Work out the finished part from the listing and answer in its coordinate system (mm). Face numbers are marked on the shaded views. A direction names the side the tool comes from. Coordinates: 2 decimals unless noted, no trailing zeros. Order: outer loops, then holes, each group sorted by start corner. A loop starts at its lowest first (then second) coordinate and runs counter-clockwise, first axis right, second up. Notation, with made-up numbers: M 81.5,9.25 L 99.5,9.25 A32 ccw 99.5,42.25 Z; hole C -20,67 d4. An arc over 180 degrees is marked long. Use a Markdown table: item, result. Add a question column.
from build123d import *

# Parameters (mm, degrees)
PAD006_DEPTH       = 6.8
POCKET007_DEPTH    = 2.101
POCKET009_DEPTH    = 2.101
CHAMFER003_SIZE    = 0.5
SKETCH023_R        = 3.125
SKETCH023_R_2      = 2
POCKET021_DEPTH    = 2.9
POCKET021_FACE36_R = 3.125
POCKET022_DEPTH    = 3.901
POCKET023_DEPTH    = 5.6
CHAMFER006_SIZE    = 0.4
SKETCH021_R        = 0.5
POCKET024_DEPTH    = 6.801
CHAMFER007_SIZE    = 1


with BuildPart() as part:
    # ShapeBinder001 → Pad006 (new body)
    with BuildSketch(Plane(origin=(0, 0, -2.55), x_dir=(0, -1, 0), z_dir=(0, 0, -1))):
        with BuildLine():
            Line((21, -17), (21, 17))
            ThreePointArc((21, 17), (19.535534, 20.535534), (16, 22))
            Line((16, 22), (-16, 22))
            ThreePointArc((-16, 22), (-19.535534, 20.535534), (-21, 17))
            Line((-21, 17), (-21, -17))
            ThreePointArc((-21, -17), (-19.535534, -20.535534), (-16, -22))
            Line((-16, -22), (16, -22))
            ThreePointArc((16, -22), (19.535534, -20.535534), (21, -17))
        make_face()
    extrude(amount=PAD006_DEPTH)

    # Sketch012 (on Face1 of ShapeBinder003) → Pocket007 (cut, through all)
    with BuildSketch(Plane(origin=(0, 0, -4.65), x_dir=(1, 0, 0), z_dir=(0, 0, -1))):
        with BuildLine():
            Line((-22, -16), (-22, -15.101687))
            Line((-22, -15.101687), (-20.818291, -15.101687))
            Line((-20.818291, -15.101687), (-3.618291, -11.901687))
            Line((-3.618291, -11.901687), (3.618291, -11.901687))
            Line((3.618291, -11.901687), (20.818291, -15.101687))
            Line((20.818291, -15.101687), (22, -15.101687))
            Line((22, -15.101687), (22, -16))
            ThreePointArc((17, -21), (20.535534, -19.535534), (22, -16))
            Line((17, -21), (-17, -21))
            ThreePointArc((-22, -16), (-20.535534, -19.535534), (-17, -21))
        make_face()
    extrude(amount=-POCKET007_DEPTH, mode=Mode.SUBTRACT)

    # Sketch014 (on Face1 of ShapeBinder004) → Pocket009 (cut, through all)
    with BuildSketch(Plane(origin=(0, 0, -4.65), x_dir=(1, 0, 0), z_dir=(0, 0, -1))):
        with BuildLine():
            Line((17, 21), (-17, 21))
            ThreePointArc((-17, 21), (-20.535534, 19.535534), (-22, 16))
            Line((-22, 14.7), (-22, 16))
            Line((-20.8, 14.7), (-22, 14.7))
            ThreePointArc((-12.754477, 12.316141), (-16.604371, 14.0915), (-20.8, 14.7))
            ThreePointArc((-12.754477, 12.316141), (-8.852447, 10.516741), (-4.6, 9.9))
            Line((-4.6, 9.9), (4.6, 9.9))
            ThreePointArc((4.6, 9.9), (8.852447, 10.516741), (12.754477, 12.316141))
            ThreePointArc((20.8, 14.7), (16.604371, 14.0915), (12.754477, 12.316141))
            Line((20.8, 14.7), (22, 14.7))
            Line((22, 14.7), (22, 16))
            ThreePointArc((22, 16), (20.535534, 19.535534), (17, 21))
        make_face()
    extrude(amount=-POCKET009_DEPTH, mode=Mode.SUBTRACT)

    # Chamfer003
    chamfer003_edges = [part.edges().sort_by_distance(p)[0] for p in [
        (-21.4, -14.7, -2.55),
        (-16.604371, -14.0915, -2.55),
        (-8.852447, -10.516741, -2.55),
        (0, -9.9, -2.55),
        (8.852447, -10.516741, -2.55),
        (16.604371, -14.0915, -2.55),
        (21.4, -14.7, -2.55),
        (22, 0.200843, -2.55),
        (21.409145, 15.101687, -2.55),
        (12.218291, 13.501687, -2.55),
        (0, 11.901687, -2.55),
        (-12.218291, 13.501687, -2.55),
        (-21.409145, 15.101687, -2.55),
        (-22, 0.200843, -2.55),
        (0, -21, -4.65),
        (0, 21, -4.65),
        (22, -14.7, -3.6),
        (-22, -14.7, -3.6),
        (22, 15.101687, -3.6),
        (-22, 15.101687, -3.6),
    ]]
    chamfer(chamfer003_edges, length=CHAMFER003_SIZE)

    # Sketch023 → Pocket021 (cut)
    with BuildSketch(Plane(origin=(0, 0, -9.35), x_dir=(1, 0, 0), z_dir=(0, 0, -1))):
        Circle(SKETCH023_R)
        with Locations((0, 14)):
            Circle(SKETCH023_R_2)
    extrude(amount=-POCKET021_DEPTH, mode=Mode.SUBTRACT)

    # Pocket021 Face36 → Pocket022 (cut, through all)
    with BuildSketch(Plane(origin=(0, 0, -6.45), x_dir=(0, -1, 0), z_dir=(0, 0, -1))):
        Circle(POCKET021_FACE36_R)
    extrude(amount=-POCKET022_DEPTH, mode=Mode.SUBTRACT)

    # Sketch024 (on Face40 of Pocket022) → Pocket023 (cut)
    with BuildSketch(Plane.XY.offset(-2.55)):
        Polygon((0, 6.466323), (-5.6, 3.233162), (-5.6, -3.233162), (0, -6.466323), (5.6, -3.233162), (5.6, 3.233162), align=None)
    extrude(amount=-POCKET023_DEPTH, mode=Mode.SUBTRACT)

    # Chamfer006
    chamfer006_edges = [part.edges().sort_by_distance(p)[0] for p in [
        (0, -21, -9.35),
        (-20.535534, -19.535534, -9.35),
        (20.535534, -19.535534, -9.35),
        (-22, 0, -9.35),
        (22, 0, -9.35),
        (-20.535534, 19.535534, -9.35),
        (20.535534, 19.535534, -9.35),
        (0, 21, -9.35),
        (-3.125, 0, -9.35),
        (-2, -14, -9.35),
    ]]
    chamfer(chamfer006_edges, length=CHAMFER006_SIZE)

    # Sketch021 (on Face38 of Chamfer003) → Pocket024 (cut, through all)
    with BuildSketch(Plane.XY.offset(-2.55)):
        with Locations((-12.8, -0.1)):
            Circle(SKETCH021_R)
        with Locations((12.8, -0.1)):
            Circle(SKETCH021_R)
    extrude(amount=-POCKET024_DEPTH, mode=Mode.SUBTRACT)

    # Chamfer007
    chamfer007_edges = [part.edges().sort_by_distance(p)[0] for p in [
        (5.6, 0, -2.55),
        (2.8, 4.849742, -2.55),
        (-2.8, 4.849742, -2.55),
        (-5.6, 0, -2.55),
        (-2.8, -4.849742, -2.55),
        (2.8, -4.849742, -2.55),
    ]]
    chamfer(chamfer007_edges, length=CHAMFER007_SIZE)


solid = part.part
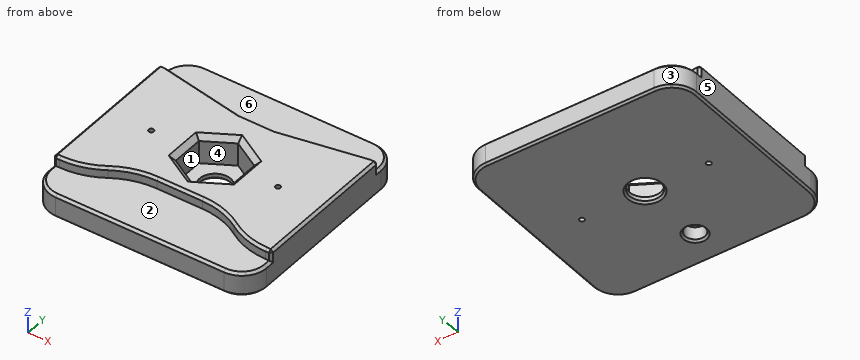
(1) Straight lines are drawn through the part: line 1 (Y direction, x = 0, z = -8.65) (3 decimals); line 2 (Y direction, x = 0, z = -6.95); line 3 (Y direction, x = -12.8, z = -7.25). For each, find the intervals that lie inside material, in ascending order.
(2) Given P1, Ø0.8, axis at x = -0.5, z = -4, coming from the +Y side; P2, Ø4.5, axis at x = 0, y = -14, coming from the -Z side; P3, Ø0.5, axis at x = 21, z = -4, coming from the +Y side, each flat-ended and moving along its own axis, determine where each tip first touches the part or whether it passes through.
(3) Which of the six approach directions +Z, -Z, +X, -X, +Y, -Y give full straight-line access (tool end or side, diameter ignored) to the marked faces 4, 5 and 6?
(4) The mould has two halves that part along Y. Classify the marked faces 1, 2 and 3: pulls with the +Y half, pulls with the -Y half, needs draft (parallel to the pull), parting line crosses it, or undercut.
(5) A cutting plane is placed at B-B on y = -5.5. Write down the section's boundary in (x, z), plus the area to 3 significant figures.
(6) A cutting plane is placed at A-A on y = 13. Write down the section's boundary in (x, z).
From the geometry:
| question | item | result |
|---|---|---|
| 1 | line 1 | y = -21 to -16, -12 to -3.125, 3.125 to 21 |
| 1 | line 2 | y = -21 to -16, -12 to -6.47, 6.47 to 21 |
| 1 | line 3 | y = -21 to -0.6, 0.4 to 21 |
| 2 | P1 | stops at y = 11.9 |
| 2 | P2 | stops at z = -9.2 |
| 2 | P3 | stops at y = 15.1 |
| 3 | face 4 | +Z |
| 3 | face 5 | +Z, -Z, -X, +Y, -Y |
| 3 | face 6 | +Z, +Y |
| 4 | face 1 | undercut |
| 4 | face 2 | needs draft |
| 4 | face 3 | pulls with the +Y half |
| 5 | outline | M -22,-8.95 L -21.6,-9.35 L 21.6,-9.35 L 22,-8.95 L 22,-3.05 L 21.5,-2.55 L 3.67,-2.55 L 1.67,-3.55 L 1.67,-8.15 L -1.67,-8.15 L -1.67,-3.55 L -3.67,-2.55 L -21.5,-2.55 L -22,-3.05 Z |
| 5 | area | 278 mm2 |
| 6 | outline | M -22,-8.95 L -21.6,-9.35 L 21.6,-9.35 L 22,-8.95 L 22,-3.05 L 21.5,-2.55 L 12.26,-2.55 L 9.52,-3.05 L 9.52,-4.65 L -9.52,-4.65 L -9.52,-3.05 L -12.26,-2.55 L -21.5,-2.55 L -22,-3.05 Z |
